```python
from build123d import *

# Parameters (mm, degrees)
IZIM1_R                     = 17
IZIM1_R_2                   = 12.5
Y_KSEKLIK_EKSTR_ZYON1_DEPTH = 34
RADYUS1_R                   = 0.5
KES_EKSTR_ZYON1_DEPTH       = 42.641325709
KES_EKSTR_ZYON1_DEPTH_BACK  = 42.641325709
IZIM2_R                     = 2.5


with BuildPart() as part:
    # Çizim1 → Yükseklik-Ekstrüzyon1 (new body)
    with BuildSketch(Plane.XY):
        Circle(IZIM1_R)
        Circle(IZIM1_R_2, mode=Mode.SUBTRACT)
    extrude(amount=Y_KSEKLIK_EKSTR_ZYON1_DEPTH)

    # Radyus1
    radyus1_edges = [part.edges().sort_by_distance(p)[0] for p in [
        (-17, 0, 0),
        (-17, 0, 34),
        (-12.5, 0, 0),
        (-12.5, 0, 34),
    ]]
    fillet(radyus1_edges, radius=RADYUS1_R)

    # Çizim2 → Kes-Ekstrüzyon1 (cut, two sides: drawn at the far end of the back side and taken through both)
    with BuildSketch(Plane(origin=(0, 0, 0), x_dir=(1, 0, 0), z_dir=(0, 1, 0)).offset(-KES_EKSTR_ZYON1_DEPTH_BACK)):
        with Locations(Location((0, -5, 0), (0, 0, 270))):
            Circle(IZIM2_R)
    extrude(amount=KES_EKSTR_ZYON1_DEPTH + KES_EKSTR_ZYON1_DEPTH_BACK, mode=Mode.SUBTRACT)


solid = part.part
```
Model file for the job. Use its own axes, mm. Coordinates: 2 decimals unless noted, no trailing zeros. Write each loop counter-clockwise with the first axis right and the second up, starting at its lowest first coordinate (ties: lowest second). Pieces come first, ordered by that corner, then holes. Notation, with made-up numbers: (84, 21) - (107, 21) arc R11 cw to (107, 27) - close; hole circle Ø3 at (28, -6). An arc over 180 degrees is marked (long way). One line per item, written item: value. Start each with the question number.
1. Flat gauge pins, fed straight in: pin 1 (8 mm diameter, centred on y = -12, z = 9, fed in from +X); pin 2 (2 mm diameter, centred on y = -8, z = 11.5, fed in from +X); pin 3 (3 mm diameter, centred on x = -12, z = 13, fed in from +Y); pin 4 (6.5 mm diameter, centred on x = 0, z = 5, fed in from -Y). Where does each tip first touch, or does it go through?
2. Slice it at B-B (x = 0). Write the cut outline in (y, z).
3. Slice it at A-A (y = 0). Write the cut outline in (x, z), plus the area to 3 significant figures.
4. Slice it at C-C (z = 4). Write the cut outline in (x, y), plus the area to 3 significant figures.
5. Mould opens along X. For faces 1 (the cylindrical face through (-3.685, -16.596, 16.769)), 2 (the flat face through (-0.1, -13.4, 34)), 3 (the cylindrical face through (5.77, -11.09, 16.77)), 4 (the cylindrical face through (0.751, 14.593, 7.385)) say: released by +X, released by -X, zero draft, split by the parting line, or undercut.
6. Slice it at D-D (z = 14). Write the cut outline in (x, y), plus the area to 3 significant figures.
7. Probe line 1 (Y direction, x = 0, z = 19); line 2 (Z direction, x = 0, y = 16); line 3 (Y direction, x = 4, z = 23). List the from-to ranges inside material, lowest first. Write a range as from..to.
Answers below:
1. pin 1: stops at x = 15
1. pin 2: stops at x = 15.49
1. pin 3: stops at y = 13.37
1. pin 4: stops at y = -17
2. outline: (-17, 0.5) arc R0.5 ccw to (-16.5, 0) - (-13, 0) arc R0.5 ccw to (-12.5, 0.5) - (-12.5, 2.5) - (-17, 2.5) - close; (-17, 7.5) - (-12.5, 7.5) - (-12.5, 33.5) arc R0.5 ccw to (-13, 34) - (-16.5, 34) arc R0.5 ccw to (-17, 33.5) - close; (12.5, 0.5) arc R0.5 ccw to (13, 0) - (16.5, 0) arc R0.5 ccw to (17, 0.5) - (17, 2.5) - (12.5, 2.5) - close; (12.5, 7.5) - (17, 7.5) - (17, 33.5) arc R0.5 ccw to (16.5, 34) - (13, 34) arc R0.5 ccw to (12.5, 33.5) - close
3. outline: (-17, 0.5) arc R0.5 ccw to (-16.5, 0) - (-13, 0) arc R0.5 ccw to (-12.5, 0.5) - (-12.5, 33.5) arc R0.5 ccw to (-13, 34) - (-16.5, 34) arc R0.5 ccw to (-17, 33.5) - close; (12.5, 0.5) arc R0.5 ccw to (13, 0) - (16.5, 0) arc R0.5 ccw to (17, 0.5) - (17, 33.5) arc R0.5 ccw to (16.5, 34) - (13, 34) arc R0.5 ccw to (12.5, 33.5) - close
3. area: 306 mm^2
4. outline: (-2.29, -16.84) - (-2.29, -12.29) arc R12.5 cw to (-2.29, 12.29) - (-2.29, 16.84) arc R17 ccw to start; (2.29, -16.84) arc R17 ccw to (2.29, 16.84) - (2.29, 12.29) arc R12.5 cw to (2.29, -12.29) - close
4. area: 376 mm^2
5. face 1: split by the parting line
5. face 2: zero draft
5. face 3: undercut
5. face 4: undercut
6. outline: circle Ø34 at (0, 0); hole circle Ø25 at (0, 0)
6. area: 417 mm^2
7. line 1: y = -17..-12.5, 12.5..17
7. line 2: z = 0..2.5, 7.5..34
7. line 3: y = -16.52..-11.84, 11.84..16.52
